Can you work these out from the model? Positions are in its coordinate system, mm. Face numbers are marked on the shaded views. A direction names the side the tool comes from. Round coordinates to 2 decimals unless told otherwise and drop trailing zeros. Order: outer loops, then holes, each group sorted by start corner. A loop starts at its lowest first (then second) coordinate and runs counter-clockwise, first axis right, second up. Notation, with made-up numbers: (17, 4.25) - (35, 4.25) arc R33 ccw to (35, 42.25) - close; hole circle Ø7 at (59, 77.25). An arc over 180 degrees is marked (long way). Write item = value, one per line.
from build123d import *

# Parameters (mm, degrees)
F0_W     = 40
F0_H     = 40
F1_DEPTH = 40


with BuildPart() as f1:
    # F0 (on Front) → F1 (new body)
    with BuildSketch(Plane.XZ):
        Polygon((0, 20), (0, 0), (60, 0), (60, 20), (50, 20), (10, 20), align=None)
        with Locations((30, 40)):
            Rectangle(F0_W, F0_H)
    extrude(amount=-F1_DEPTH)


solid = f1.part
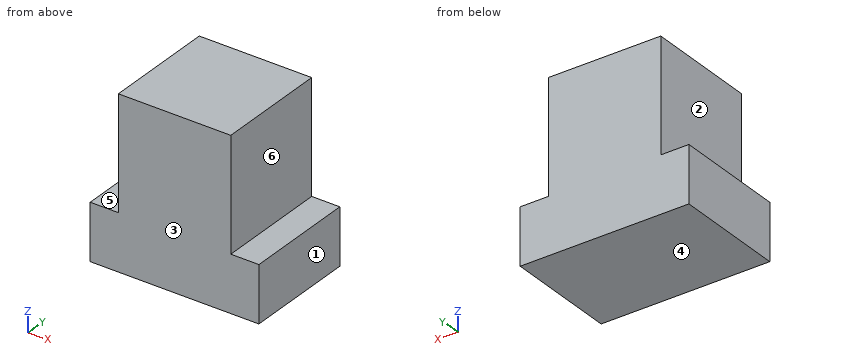
(1) Thinking about a two-plate mould opening in X: for the marked faces 1, 2 and 3, which applies, +X half, -X half, draft (parallel to the pull), parting line (faces both ways), or undercut?
Computed:
face_1 = +X half
face_2 = -X half
face_3 = draft
(2) If we section it at B-B (z = 53): Write out the boundary of the cut face in (x, y).
Computed:
outline = (10, 0) - (50, 0) - (50, 40) - (10, 40) - close
(3) If I drill on line 1 (Z direction, x = 54.5, y = 14); line 2 (X direction, y = 28, z = 28.5), over which ranges is the centre line in solid material (lowest first)? Write a range as from..to.
Computed:
line_1 = 0..20
line_2 = 10..50
(4) If we section it at A-A (y = 31): Write out the boundary of the cut face in (x, z), plus the area to 3 significant figures.
Computed:
outline = (0, 0) - (60, 0) - (60, 20) - (50, 20) - (50, 60) - (10, 60) - (10, 20) - (0, 20) - close
area = 2,800 mm^2
(5) Will these pins go through, and if not, where does the flat tip stop? P1, Ø3, axis at y = 35.5, z = 49, coming from the +X side; P2, Ø3, axis at x = 53, y = 18, coming from the +Z side; P3, Ø12, axis at y = 23, z = 32.5, coming from the -X side.
Computed:
P1 = 50
P2 = 20
P3 = 10
(6) If we section it at C-C (x = 4.5): Write out the boundary of the cut face in (y, z).
Computed:
outline = (0, 0) - (40, 0) - (40, 20) - (0, 20) - close
(7) On a 3-axis mill with a long thin cutter (end or side, diameter ignored), from which of +Z, -Z, +X, -X, +Y, -Y can I reach the whole of each face in a straight line? I mean the marked faces 4, 5 and 6. Say none if no direction works.
Computed:
face_4 = -Z, +X, -X, +Y, -Y
face_5 = +Z, -X, +Y, -Y
face_6 = +Z, +X, +Y, -Y
